from build123d import *

# Parameters (mm, degrees)
BOSS_EXTRUDE2_DEPTH = 4
CUT_EXTRUDE1_DEPTH  = 5


with BuildPart() as part:
    # Sketch1 → Boss-Extrude2 (new body)
    with BuildSketch(Plane.XY):
        with BuildLine():
            Line((-19.985447982, 0.762803358), (-59.956343946, 2.288410074))
            ThreePointArc((-59.956343946, 2.288410074), (-55.730717245, 22.228071336), (-45.073672701, 39.602576043))
            Line((-45.073672701, 39.602576043), (-13.592462366, 14.67122922))
            ThreePointArc((-13.592462366, 14.67122922), (-18.172234131, 8.352838241), (-19.985447982, 0.762803358))
        make_face()
    extrude(amount=BOSS_EXTRUDE2_DEPTH)

    # Sketch1_5 → Cut-Extrude1 (cut, through all)
    with BuildSketch(Plane.XY):
        with BuildLine():
            ThreePointArc((-19.494667642, 10.19597634), (-20.144482043, 8.843067523), (-20.700540486, 7.449001516))
            Line((-20.700540486, 7.449001516), (-55.106686022, 18.090139737))
            ThreePointArc((-55.106686022, 18.090139737), (-54.275723264, 20.448615214), (-53.343874365, 22.769081398))
            Line((-53.343874365, 22.769081398), (-19.494667642, 10.19597634))
        make_face()
        with BuildLine():
            Line((-21.2282638, 5.775882272), (-57.269563461, 9.175897829))
            ThreePointArc((-57.269563461, 9.175897829), (-57.611850796, 6.698854216), (-57.847050894, 4.209358967))
            Line((-57.847050894, 4.209358967), (-21.816681027, 2.834154011))
            ThreePointArc((-21.816681027, 2.834154011), (-21.572673921, 4.315059664), (-21.2282638, 5.775882272))
        make_face()
        with BuildLine():
            ThreePointArc((-16.356919422, 14.712280144), (-17.245912522, 13.659374118), (-18.067243214, 12.552877066))
            Line((-18.067243214, 12.552877066), (-48.546898537, 31.736393028))
            ThreePointArc((-48.546898537, 31.736393028), (-47.133831778, 33.799436415), (-45.633154018, 35.799654388))
            Line((-45.633154018, 35.799654388), (-16.19149009, 14.894148135))
            Line((-16.19149009, 14.894148135), (-16.356919422, 14.712280144))
        make_face()
    extrude(amount=CUT_EXTRUDE1_DEPTH, mode=Mode.SUBTRACT)


solid = part.part
Work out the finished part from the listing and answer in its coordinate system (mm). A direction names the side the tool comes from. Give positions to 0.01 mm unless a question says otherwise; leave off trailing zeros. Loops run counter-clockwise (first coordinate to the right, second up) from the corner with the lowest first, then second, coordinate; pieces in that order, holes last. Notation, with made-up numbers: (53.5, 21) -> (72.5, 21) arc R17 ccw to (72.5, 51) -> close; hole circle Ø6 at (32.25, -33.5). An arc over 180 degrees is marked (long way). Use a Markdown table: item, result. Add a question column.
1. For faces 4 (the flat face through (-42, 12, 4)), 5 (the cylindrical face through (-47.154, 33.771, 1.972)), determine the directions among +Z, -Z, +X, -X, +Y, -Y from which every point of the face is accessible in a straight line to the end or side of a thin tool.
2. Find the intervals of material crossed by probe 1 along Y at (x, z) = (-47.5, 1.1); probe 2 along Y at (x, z) = (-45.5, 2.05); probe 3 along Y at (x, z) = (-53.5, 0.4), in increasing order.
3. Section C-C on x = -24.5 is taken. Determine the outline of the cut face in (y, z).
4. Flat-ended cylindrical pins translate along their axes: pin 1 Ø2 at (x, z) = (-51, 2.5) entering from +Y; pin 2 Ø1.5 at (x, z) = (-30, 2.5) entering from +Y; pin 3 Ø1 at (x, z) = (-26, 1.5) entering from -Y. Find the tip coordinate at first contact, or state that the pin passes through.
5. Determine the mould class of faces 1 (the flat face through (-33.09, 22.01, 1.97)), 2 (the flat face through (-42, 12, 0)), 3 (the cylindrical face through (-55.836, 21.961, 1.972)) for opening direction X: released by +X, released by -X, zero draft, split by the parting line, or undercut.
6. Section B-B on y = 5 is taken. Determine the outline of the cut face in (x, z).
7. Section A-A on z = 2.55 is taken. Determine the outline of the cut face in (x, y), and give its area (3 significant figures).
8. Section D-D on y = 16.5 is taken. Determine the outline of the cut face in (x, z).
Results below:
| question | item | result |
|---|---|---|
| 1 | face 4 | +Z, +X, -X, +Y, -Y |
| 1 | face 5 | +Z, -Z |
| 2 | probe 1 | y = 1.81 to 3.81, 8.25 to 15.74, 20.6 to 31.08, 33.28 to 36.66 |
| 2 | probe 2 | y = 1.74 to 3.74, 8.07 to 15.12, 19.86 to 29.82, 35.71 to 39.11 |
| 2 | probe 3 | y = 2.04 to 4.04, 8.82 to 17.59, 22.4 to 27.16 |
| 3 | outline | (0.94, 0) -> (2.94, 0) -> (2.94, 4) -> (0.94, 4) -> close; (6.08, 0) -> (8.62, 0) -> (8.62, 4) -> (6.08, 4) -> close; (12.06, 0) -> (16.6, 0) -> (16.6, 4) -> (12.06, 4) -> close; (20.79, 0) -> (23.31, 0) -> (23.31, 4) -> (20.79, 4) -> close |
| 4 | pin 1 | stops at y = 33.17 |
| 4 | pin 2 | stops at y = 28.26 |
| 4 | pin 3 | stops at y = 0.97 |
| 5 | face 1 | undercut |
| 5 | face 2 | zero draft |
| 5 | face 3 | released by -X |
| 6 | outline | (-59.79, 0) -> (-57.78, 0) -> (-57.78, 4) -> (-59.79, 4) -> close; (-21.42, 0) -> (-19.36, 0) -> (-19.36, 4) -> (-21.42, 4) -> close |
| 7 | outline | (-59.96, 2.29) -> (-19.99, 0.76) arc R20 cw to (-13.59, 14.67) -> (-45.07, 39.6) arc R60 ccw to start; hole (-57.85, 4.21) -> (-21.82, 2.83) arc R22 cw to (-21.23, 5.78) -> (-57.27, 9.18) arc R58 ccw to start; hole (-55.11, 18.09) -> (-20.7, 7.45) arc R22 cw to (-19.49, 10.2) -> (-53.34, 22.77) arc R58 ccw to start; hole (-48.55, 31.74) -> (-18.07, 12.55) arc R22 cw to (-16.36, 14.71) -> (-16.19, 14.89) -> (-45.63, 35.8) arc R58 ccw to start |
| 7 | area | 701 mm^2 |
| 8 | outline | (-57.69, 0) -> (-49.97, 0) -> (-49.97, 4) -> (-57.69, 4) -> close; (-36.47, 0) -> (-24.34, 0) -> (-24.34, 4) -> (-36.47, 4) -> close; (-18.45, 0) -> (-15.9, 0) -> (-15.9, 4) -> (-18.45, 4) -> close |
